Geometry check sheet. Reference: the model listing, model coordinates, mm. A direction names the side the tool comes from. Round coordinates to 2 decimals unless told otherwise and drop trailing zeros. Order: outer loops, then holes, each group sorted by start corner. A loop starts at its lowest first (then second) coordinate and runs counter-clockwise, first axis right, second up.
(1) Set-up check for faces 4 (the face through (12.359, -30.2, -30.2)), 5 (the face through (25.254, -34.788, -7.725)), 6 (the face through (2.989, -34.788, -7.725)): record each of +Z, -Z, +X, -X, +Y, -Y from which the full face is reachable in a straight line by a thin tool's end or side.
(2) Cross-section at D-D on y = -37.5. Enter the section's corners in (x, z).
(3) Thickness scan on L1, parallel to Y at x = 6.25, z = 0; L2, parallel to X at y = 29, z = 33; L3, parallel to Y at x = 5, z = 0. Record the ranges inside material, lowest first.
(4) Gauge pin test, flat ends, axial feed: P1, Ø1, axis at y = 17.5, z = -0.5, coming from the +X side; P2, Ø1.5, axis at x = 27, z = 26, coming from the +Y side; P3, Ø2, axis at y = -22.5, z = -1, coming from the +X side; P4, Ø1, axis at y = -20.5, z = 2, coming from the -X side. Record the tip position at first contact, or that the pin passes through.
(5) Cross-section at C-C on z = 37. Enter the section's corners in (x, y).
(6) Draft check along Y on faces 1 (the face through (9.2, -44.5, -9.9)), 2 (the face through (22.618, -23.4, 27.2)), 3 (the face through (14.456, 0, -6)). Enter one of: pulls with the +Y half, pulls with the -Y half, needs draft (parallel to the pull), parting line crosses it, or undercut.
from build123d import *


with BuildPart() as f1:
    # F0 (on Front) → F1 (revolve)
    with BuildSketch(Plane.XZ):
        with BuildLine():
            Line((0, 35.635482), (0, 0))
            Line((0, 0), (54.456629, 0))
            Line((54.456629, 0), (54.456629, 9.35728))
            ThreePointArc((54.456629, 9.35728), (37.055172, 18.307365), (27.963908, 35.635482))
            Line((27.963908, 35.635482), (22.618492, 35.635482))
            Line((22.618492, 35.635482), (22.618492, 45.586757))
            Line((22.618492, 45.586757), (15.856263, 45.586757))
            Line((15.856263, 45.586757), (15.856263, 42.555407))
            Line((15.856263, 42.555407), (12.358558, 42.555407))
            Line((12.358558, 42.555407), (12.358558, 45.586757))
            Line((12.358558, 45.586757), (6.062689, 45.586757))
            Line((6.062689, 45.586757), (6.062689, 35.635482))
            Line((6.062689, 35.635482), (0, 35.635482))
        make_face()
    revolve(axis=Axis((27.228314, 0, 0), (-1, 0, 0)))

    # F2 (on Front) → F3 (revolve, cut)
    with BuildSketch(Plane.XZ):
        Polygon((0, 13.247386), (0, 0), (56.932209, 0), (56.932209, 4.994054), (14.45647, 4.994054), (14.45647, 13.247386), align=None)
    revolve(axis=Axis((28.466105, 0, 0), (-1, 0, 0)), mode=Mode.SUBTRACT)


solid = f1.part
Found:
1. face 4: none
1. face 5: +X
1. face 6: -X
2. outline: (6.06, -25.92) - (12.36, -25.92) - (12.36, -20.12) - (15.86, -20.12) - (15.86, -25.92) - (22.62, -25.92) - (22.62, 25.92) - (15.86, 25.92) - (15.86, 20.12) - (12.36, 20.12) - (12.36, 25.92) - (6.06, 25.92) - close
3. L1: y = -45.59 to -13.25, 13.25 to 45.59
3. L2: x = 6.06 to 12.36, 15.86 to 22.62
3. L3: y = -35.64 to -13.25, 13.25 to 35.64
4. P1: stops at x = 38.45
4. P2: stops at y = 25.15
4. P3: stops at x = 34.22
4. P4: stops at x = 0
5. outline: (6.06, -26.63) - (12.36, -26.63) - (12.36, -21.02) - (15.86, -21.02) - (15.86, -26.63) - (22.62, -26.63) - (22.62, 26.63) - (15.86, 26.63) - (15.86, 21.02) - (12.36, 21.02) - (12.36, 26.63) - (6.06, 26.63) - close
6. face 1: parting line crosses it
6. face 2: needs draft
6. face 3: undercut
